```python
from build123d import *

# Parameters (mm, degrees)
SKETCH_1_W      = 17
SKETCH_1_H      = 16
SKETCH_1_R      = 1
SKETCH_1_R_2    = 4
EXTRUDE_1_DEPTH = 4
FILLET_1_R      = 1


with BuildPart() as part:
    # 草图1 → 凸台-拉伸1 (new body)
    with BuildSketch(Plane(origin=(0, 0, 0), x_dir=(1, 0, 0), z_dir=(0, 1, 0))):
        Rectangle(SKETCH_1_W, SKETCH_1_H)
        with Locations(Location((6, 4, 0), (0, 0, 270))):
            Circle(SKETCH_1_R, mode=Mode.SUBTRACT)
        with Locations(Location((-6, 4, 0), (0, 0, 90))):
            Circle(SKETCH_1_R, mode=Mode.SUBTRACT)
        with Locations(Location((6, -4, 0), (0, 0, 90))):
            Circle(SKETCH_1_R, mode=Mode.SUBTRACT)
        with Locations(Location((-6, -4, 0), (0, 0, 270))):
            Circle(SKETCH_1_R, mode=Mode.SUBTRACT)
        with Locations(Location((0, 0, 0), (0, 0, 270))):
            Circle(SKETCH_1_R_2, mode=Mode.SUBTRACT)
    extrude(amount=EXTRUDE_1_DEPTH)

    # 圆角1
    fillet_1_edges = [part.edges().sort_by_distance(p)[0] for p in [
        (8.5, 2, 8),
        (-8.5, 2, 8),
        (-8.5, 2, -8),
        (8.5, 2, -8),
    ]]
    fillet(fillet_1_edges, radius=FILLET_1_R)


solid = part.part
```
Input: part model. Units: mm. Frame: model coordinates. Round coordinates to 2 decimals unless told otherwise and drop trailing zeros. Order: outer loops, then holes, each group sorted by start corner. A loop starts at its lowest first (then second) coordinate and runs counter-clockwise, first axis right, second up. Notation, with made-up numbers: (15, 55) - (49, 55) arc R24 ccw to (49, 68) - close; hole circle Ø3 at (-7, 5.5). An arc over 180 degrees is marked (long way). Answer in a Markdown table with one row per item.
Item 1: Section query D-D (x = -6). Return the cut outline in (y, z), then the cut area to 3 significant figures.
Model answer:
| item | result |
|---|---|
| outline | (0, -8) - (4, -8) - (4, -5) - (0, -5) - close; (0, -3) - (4, -3) - (4, 3) - (0, 3) - close; (0, 5) - (4, 5) - (4, 8) - (0, 8) - close |
| area | 48.0 mm² |
Item 2: Mould query, pull axis X, two halves, no side actions, for faces 1 (the cylindrical face through (-5.324, 1.972, 3.263)), 2 (the flat face through (8.5, 2, 0)), 3 (the flat face through (0, 2, 8)). Classes: released by +X, released by -X, zero draft, split by the parting line, or undercut.
Model answer:
| item | result |
|---|---|
| face 1 | undercut |
| face 2 | released by +X |
| face 3 | zero draft |
Item 3: Pin query (flat end, axial travel): pin 1 (1.6 mm diameter, centred on x = -6, z = 4, fed in from +Y); pin 2 (3 mm diameter, centred on x = -6.5, z = -4, fed in from +Y). Return the tip coordinate at first contact, or that it passes through.
Model answer:
| item | result |
|---|---|
| pin 1 | passes through |
| pin 2 | stops at y = 4 |
Item 4: Section query B-B (y = 0.65). Return the cut outline in (x, z), then the cut area to 3 significant figures.
Model answer:
| item | result |
|---|---|
| outline | (-8.5, -7) arc R1 ccw to (-7.5, -8) - (7.5, -8) arc R1 ccw to (8.5, -7) - (8.5, 7) arc R1 ccw to (7.5, 8) - (-7.5, 8) arc R1 ccw to (-8.5, 7) - close; hole circle Ø2 at (-6, -4); hole circle Ø2 at (-6, 4); hole circle Ø8 at (0, 0); hole circle Ø2 at (6, -4); hole circle Ø2 at (6, 4) |
| area | 208 mm² |
Item 5: Line query: line 1 (X direction, y = 2.55, z = 3.25); line 2 (Z direction, x = 5.25, y = 3.6); line 3 (X direction, y = 3.5, z = -4.75). Output: solid intervals per line, ascending.
Model answer:
| item | result |
|---|---|
| line 1 | x = -8.5 to -6.66, -5.34 to -2.33, 2.33 to 5.34, 6.66 to 8.5 |
| line 2 | z = -8 to -4.66, -3.34 to 3.34, 4.66 to 8 |
| line 3 | x = -8.5 to -6.66, -5.34 to 5.34, 6.66 to 8.5 |
Item 6: Section query A-A (x = 0). Return the cut outline in (y, z).
Model answer:
| item | result |
|---|---|
| outline | (0, -8) - (4, -8) - (4, -4) - (0, -4) - close; (0, 4) - (4, 4) - (4, 8) - (0, 8) - close |
Item 7: Section query C-C (z = 0). Return the cut outline in (x, y), then the cut area to 3 significant figures.
Model answer:
| item | result |
|---|---|
| outline | (-8.5, 0) - (-4, 0) - (-4, 4) - (-8.5, 4) - close; (4, 0) - (8.5, 0) - (8.5, 4) - (4, 4) - close |
| area | 36.0 mm² |
